```python
from build123d import *

# Parameters (mm, degrees)
F0_W     = 115
F0_H     = 10
F1_DEPTH = 10
F2_W     = 15
F2_H     = 10
F3_DEPTH = 5
F4_W     = 25
F4_H     = 10
F5_DEPTH = 2.5


with BuildPart() as f1:
    # F0 (on Front) → F1 (new body)
    with BuildSketch(Plane.XZ):
        with Locations((0, -5)):
            Rectangle(F0_W, F0_H)
    extrude(amount=F1_DEPTH)

    # F2 (on face) → F3 (cut)
    with BuildSketch(Plane.XY):
        with Locations((50, -5)):
            Rectangle(F2_W, F2_H)
    extrude(amount=-F3_DEPTH, mode=Mode.SUBTRACT)

    # F4 (on face) → F5 (join)
    with BuildSketch(Plane(origin=(0, 0, -10), x_dir=(1, 0, 0), z_dir=(0, 0, -1))):
        with Locations((-65, 5)):
            Rectangle(F4_W, F4_H)
    extrude(amount=F5_DEPTH)


solid = f1.part
```
Input: part model. Units: mm. Frame: model coordinates. A direction names the side the tool comes from. Give positions to 0.01 mm unless a question says otherwise; leave off trailing zeros. Order: outer loops, then holes, each group sorted by start corner. A loop starts at its lowest first (then second) coordinate and runs counter-clockwise, first axis right, second up.
1. Cut plane B-B (x = 7). Return loops of the section in (y, z).
Computed:
outline: (-10, -10) - (0, -10) - (0, 0) - (-10, 0) - close
2. Cut plane C-C (z = -6.75). Return loops of the section in (x, y).
Computed:
outline: (-57.5, -10) - (57.5, -10) - (57.5, 0) - (-57.5, 0) - close
3. Cut plane A-A (y = -2.25). Return loops of the section in (x, z), and give its area (3 significant figures).
Computed:
outline: (-77.5, -12.5) - (-52.5, -12.5) - (-52.5, -10) - (57.5, -10) - (57.5, -5) - (42.5, -5) - (42.5, 0) - (-57.5, 0) - (-57.5, -10) - (-77.5, -10) - close
area: 1,140 mm2
4. Set-up query: faces 1 (the face through (-57.5, -5, -5)), 2 (the face through (-8, -5, 0)), 3 (the face through (2, -5, -10)), 4 (the face through (42.5, -5, -2)). Return all of +Z, -Z, +X, -X, +Y, -Y with unobstructed straight access to the full face (end or side cutting, diameter ignored); none if empty.
Computed:
face 1: +Z, -X, +Y, -Y
face 2: +Z, +X, -X, +Y, -Y
face 3: -Z, +X, +Y, -Y
face 4: +Z, +X, +Y, -Y
5. Line query: probe 1 along Z at (x, y) = (24, -7.5); probe 2 along X at (y, z) = (-6.5, -2.25); probe 3 along X at (y, z) = (-1.25, -8). Output: solid intervals per line, ascending.
Computed:
probe 1: z = -10 to 0
probe 2: x = -57.5 to 42.5
probe 3: x = -57.5 to 57.5
6. Pin query (flat end, axial travel): pin 1 Ø3 at (x, y) = (-69.5, -4) entering from +Z; pin 2 Ø1.5 at (y, z) = (-5.5, -1.5) entering from +X; pin 3 Ø5 at (y, z) = (-4, -5.5) entering from -X. Return the tip coordinate at first contact, or that it passes through.
Computed:
pin 1: stops at z = -10
pin 2: stops at x = 42.5
pin 3: stops at x = -57.5
